```python
from build123d import *

# Parameters (mm, degrees)
BOSS_EXTRUDE1_DEPTH = 0.425
SKETCH2_W           = 2.75
SKETCH2_H           = 2.75
BOSS_EXTRUDE2_DEPTH = 0.1
BOSS_EXTRUDE3_START = -0.95
SKETCH3_R           = 1.025
SKETCH3_R_2         = 0.845
SKETCH3_R_3         = 0.225
BOSS_EXTRUDE3_DEPTH = 2.12
FILLET1_R           = 0.2
BOSS_EXTRUDE4_START = -0.85
SKETCH4_W           = 9.9
SKETCH4_H           = 12.5
BOSS_EXTRUDE4_DEPTH = 1.7
BOSS_EXTRUDE5_START = -0.85
SKETCH5_W           = 9.9
SKETCH5_H           = 11.125
BOSS_EXTRUDE5_DEPTH = 1.7


with BuildPart() as part:
    # Sketch1 → Boss-Extrude1 (new body, symmetric)
    with BuildSketch(Plane(origin=(0, 0, 0), x_dir=(1, 0, 0), z_dir=(0, 1, 0))):
        with BuildLine():
            Line((-5.45, -6.75), (-1.35, -6.75))
            ThreePointArc((-1.35, -6.75), (-0.642893219, -7.042893219), (-0.35, -7.75))
            Line((-0.35, -7.75), (-0.35, -8.35))
            Line((-0.35, -8.35), (5.45, -8.35))
            Line((5.45, -8.35), (5.45, -6.75))
            Line((5.45, -6.75), (5.45, 6.75))
            Line((5.45, 6.75), (-5.45, 6.75))
            Line((-5.45, 6.75), (-5.45, -6.75))
        make_face()
    extrude(amount=BOSS_EXTRUDE1_DEPTH, both=True)

    # Sketch2 → Boss-Extrude2 (add)
    with BuildSketch(Plane(origin=(0, 0.425, 0), x_dir=(1, 0, 0), z_dir=(0, 1, 0))):
        with Locations((2.55, -6.75)):
            Rectangle(SKETCH2_W, SKETCH2_H)
    extrude(amount=BOSS_EXTRUDE2_DEPTH)

    # Sketch3 → Boss-Extrude3 (add)
    with BuildSketch(Plane(origin=(0, 0.525, 0), x_dir=(1, 0, 0), z_dir=(0, 1, 0)).offset(BOSS_EXTRUDE3_START)):
        with Locations((2.55, -6.75)):
            Circle(SKETCH3_R)
        with Locations((2.55, -6.75)):
            Circle(SKETCH3_R_2, mode=Mode.SUBTRACT)
        with Locations((2.55, -6.75)):
            Circle(SKETCH3_R_3)
    extrude(amount=BOSS_EXTRUDE3_DEPTH)

    # Fillet1
    fillet1_edges = [part.edges().sort_by_distance(p)[0] for p in [
        (2.325, 1.695, 6.75),
    ]]
    fillet(fillet1_edges, radius=FILLET1_R)

    # Sketch4 → Boss-Extrude4 (add)
    with BuildSketch(Plane.XZ.offset(0.425).offset(BOSS_EXTRUDE4_START)):
        Rectangle(SKETCH4_W, SKETCH4_H)
    extrude(amount=BOSS_EXTRUDE4_DEPTH)

    # Sketch5 → Boss-Extrude5 (add)
    with BuildSketch(Plane(origin=(0, 0.425, 0), x_dir=(1, 0, 0), z_dir=(0, 1, 0)).offset(BOSS_EXTRUDE5_START)):
        with Locations((0, 0.6875)):
            Rectangle(SKETCH5_W, SKETCH5_H)
    extrude(amount=BOSS_EXTRUDE5_DEPTH)


solid = part.part
```
Work out the finished part from the listing and answer in its coordinate system (mm). A direction names the side the tool comes from. Give positions to 0.01 mm unless a question says otherwise; leave off trailing zeros. Write each loop counter-clockwise with the first axis right and the second up, starting at its lowest first coordinate (ties: lowest second). Pieces come first, ordered by that corner, then holes.
(1) The mould has two halves that part along Z. Classify faces 1 (the flat face through (3, 0.525, 7)), 2 (the flat face through (-5.45, 0, 0)), 3 (the flat face through (0, -1, -6.25)): pulls with the +Z half, pulls with the -Z half, needs draft (parallel to the pull), parting line crosses it, or undercut.
Final values:
face 1: undercut
face 2: needs draft
face 3: pulls with the -Z half
(2) Straight lines are drawn through the part: line 1 (Z direction, x = 2.55, y = 1.15) (3 decimals); line 2 (X direction, y = 1.25, z = 6.75) (3 decimals); line 3 (Y direction, x = 3.25, z = 3.25) (3 decimals). For each, find the intervals that lie inside material, in ascending order.
Final values:
line 1: z = -6.25 to 4.875, 5.725 to 5.905, 6.525 to 6.975, 7.595 to 7.775
line 2: x = 1.525 to 1.705, 2.325 to 2.775, 3.395 to 3.575
line 3: y = -1.275 to 1.275
(3) The part is cut by section B-B on y = -0.25. Write down the section's boundary in (x, z).
Final values:
outline: (-5.45, -6.75) - (5.45, -6.75) - (5.45, 8.35) - (-0.35, 8.35) - (-0.35, 7.75) arc R1 cw to (-1.35, 6.75) - (-5.45, 6.75) - close
(4) Which of the six approach directions +Z, -Z, +X, -X, +Y, -Y give full straight-line access (tool end or side, diameter ignored) to faces 4 (the flat face through (4.95, -1, 0)), 5 (the flat face through (0, 1, -6.25)), 6 (the flat face through (-3, 0, 6.75))?
Final values:
face 4: +Z, -Z, +X, -Y
face 5: -Z, +X, -X, +Y
face 6: +Z, -X, +Y, -Y
(5) Flat-ended cylindrical pins translate along their axes: pin 1 Ø0.7 at (x, y) = (-0.5, 1) entering from +Z (3 decimals); pin 2 Ø0.7 at (y, z) = (1, 0) entering from -X; pin 3 Ø0.9 at (y, z) = (1, -2.5) entering from +X. Find the tip coordinate at first contact, or state that the pin passes through.
Final values:
pin 1: stops at z = 4.875
pin 2: stops at x = -4.95
pin 3: stops at x = 4.95
(6) The part is cut by section C-C on z = -3.5. Write down the section's boundary in (x, y) (3 decimals).
Final values:
outline: (-5.45, -0.425) - (-4.95, -0.425) - (-4.95, -1.275) - (4.95, -1.275) - (4.95, -0.425) - (5.45, -0.425) - (5.45, 0.425) - (4.95, 0.425) - (4.95, 1.275) - (-4.95, 1.275) - (-4.95, 0.425) - (-5.45, 0.425) - close
(7) The part is cut by section D-D on x = 3. Write down the section's boundary in (y, z) (3 decimals).
Final values:
outline: (-1.275, -6.25) - (-0.425, -6.25) - (-0.425, -6.75) - (0.425, -6.75) - (0.425, -6.25) - (1.275, -6.25) - (1.275, 4.875) - (0.425, 4.875) - (0.425, 5.375) - (0.525, 5.375) - (0.525, 5.829) - (1.695, 5.829) - (1.695, 6.035) - (0.525, 6.035) - (0.525, 7.465) - (1.695, 7.465) - (1.695, 7.671) - (0.525, 7.671) - (0.525, 8.125) - (0.425, 8.125) - (0.425, 8.35) - (-0.425, 8.35) - (-0.425, 6.25) - (-1.275, 6.25) - close
(8) The part is cut by section A-A on x = 4.25. Write down the section's boundary in (y, z) (3 decimals).
Final values:
outline: (-1.275, -6.25) - (-0.425, -6.25) - (-0.425, -6.75) - (0.425, -6.75) - (0.425, -6.25) - (1.275, -6.25) - (1.275, 4.875) - (0.425, 4.875) - (0.425, 8.35) - (-0.425, 8.35) - (-0.425, 6.25) - (-1.275, 6.25) - close
